Part model, mm, in its own coordinate system. A direction names the side the tool comes from. Round coordinates to 2 decimals unless told otherwise and drop trailing zeros. Order: outer loops, then holes, each group sorted by start corner. A loop starts at its lowest first (then second) coordinate and runs counter-clockwise, first axis right, second up. Notation, with made-up numbers: M 5.25,-18 L 32.25,-18 A29 cw 32.25,21 Z; hole C 30,61.25 d2. An arc over 180 degrees is marked long. Write each question's results on one line, items separated by ' | '. Start each with the question number.
1. Band-saw the part on A-A, the plane y = 12. List the corners of the cut face in (x, z).
2. Band-saw the part on C-C, the plane z = 49.5. List the corners of the cut face in (x, y), then the cut area to 3 significant figures.
3. Band-saw the part on B-B, the plane x = -23.5. List the corners of the cut face in (y, z), then the cut area to 3 significant figures.
4. Band-saw the part on D-D, the plane y = -4.5. List the corners of the cut face in (x, z).
5. Which spindle directions (+Z, -Z, +X, -X, +Y, -Y) get a long thin tool onto all of the face, cutting with end or side? Do faces 4 (the face through (-2, 12, 5)), 5 (the face through (-30.753, 6, 20)). Say none if no direction does.
6. Probe L1, parallel to Z at x = 9, y = -0.5; L2, parallel to Z at x = 13, y = 6.5; L3, parallel to Y at x = -3.5, z = 55. List the from-to ranges inside material, lowest first. Write a range as [from, to].
7. Two-plate mould, pull along Z, no slides. Class faces 1 (the face through (-1.6, 7.54, 29.15)), 2 (the face through (26.747, 6, 20)), 3 (the face through (-1.6, 11.84, 26.57)): +Z half, -Z half, draft (parallel to the pull), parting line (faces both ways), or undercut.
8. Drop flat-ended pins along their axis: pin 1 Ø8 at (x, y) = (12, 4) entering from +Z; pin 2 Ø1.5 at (y, z) = (-3.5, 14.5) entering from +X; pin 3 Ø10 at (x, y) = (-22, 4.5) entering from +Z; pin 4 Ø3 at (x, z) = (-24.5, 31.5) entering from +Y. Give the stop position or say it passes through.
```python
from build123d import *

# Parameters (mm, degrees)
SKETCH3_W           = 57.5
SKETCH3_H           = 40
BOSS_EXTRUDE1_DEPTH = 57.5
CUT_EXTRUDE1_DEPTH  = 86.766124704
CUT_EXTRUDE2_DEPTH  = 86.766124704


with BuildPart() as part:
    # Sketch3 → Boss-Extrude1 (new body)
    with BuildSketch(Plane.XY):
        with Locations((-2.002808989, 7.264044944)):
            Rectangle(SKETCH3_W, SKETCH3_H)
    extrude(amount=BOSS_EXTRUDE1_DEPTH)

    # Sketch7 → Cut-Extrude1 (cut, through all)
    with BuildSketch(Plane(origin=(26.747191011, 0, 0), x_dir=(0, 0, -1), z_dir=(1, 0, 0))):
        Polygon((-57.5, 27.264044944), (0, -12.735955056), (-57.5, -12.735955056), align=None)
    extrude(amount=-CUT_EXTRUDE1_DEPTH, mode=Mode.SUBTRACT)

    # Sketch8 → Cut-Extrude2 (cut, through all)
    with BuildSketch(Plane(origin=(26.747191011, 0, 0), x_dir=(0, 0, -1), z_dir=(1, 0, 0))):
        Polygon((-5, 27.264044944), (-5, -3.166856914), (-48.744421421, 27.264044944), align=None)
    extrude(amount=-CUT_EXTRUDE2_DEPTH, mode=Mode.SUBTRACT)


solid = part.part
```
Solution:
1) outline: M -30.75,0 L 26.75,0 L 26.75,5 L -30.75,5 Z; M -30.75,26.8 L 26.75,26.8 L 26.75,35.56 L -30.75,35.56 Z
2) outline: M -30.75,21.7 L 26.75,21.7 L 26.75,27.26 L -30.75,27.26 Z | area: 320 mm^2
3) outline: M -12.74,0 L 27.26,0 L 27.26,5 L -3.17,5 L 27.26,48.74 L 27.26,57.5 Z | area: 484 mm^2
4) outline: M -30.75,0 L 26.75,0 L 26.75,11.84 L -30.75,11.84 Z
5) face 4: +X, -X, +Y | face 5: +Z, -Z, -X, +Y, -Y
6) L1: [0, 5], [8.83, 17.59] | L2: [0, 5], [18.9, 27.65] | L3: [25.52, 27.26]
7) face 1: +Z half | face 2: draft | face 3: undercut
8) pin 1: z = 29.81 | pin 2: x = 26.75 | pin 3: z = 31.96 | pin 4: y = 16.31
